```python
from build123d import *

# Parameters (mm, degrees)
BOSS_EXTRUDE1_DEPTH         = 50.8
FILLET1_R                   = 19.05
FILLET3_R                   = 3.81
F_1_4_20_TAPPED_HOLE1_D     = 5.1054
F_1_4_20_TAPPED_HOLE1_DEPTH = 19.05
F_1_4_20_TAPPED_HOLE1_TIP   = 1.533816902
M3_CLEARANCE_HOLE2_D        = 3.4


with BuildPart() as part:
    # Sketch1 → Boss-Extrude1 (new body)
    with BuildSketch(Plane.XY):
        Polygon((-20.6375, 0), (20.6375, 0), (20.6375, 6.35), (20.6375, 31.75), (12.7, 31.75), (12.7, 6.35), (-12.7, 6.35), (-12.7, 31.75), (-20.6375, 31.75), (-20.6375, 6.35), align=None)
    extrude(amount=BOSS_EXTRUDE1_DEPTH)

    # Fillet1
    fillet1_edges = [part.edges().sort_by_distance(p)[0] for p in [
        (-16.66875, 31.75, 0),
        (16.66875, 31.75, 50.8),
        (16.66875, 31.75, 0),
        (-16.66875, 31.75, 50.8),
    ]]
    fillet(fillet1_edges, radius=FILLET1_R)

    # Fillet3
    fillet3_edges = [part.edges().sort_by_distance(p)[0] for p in [
        (-12.7, 6.35, 25.4),
        (12.7, 6.35, 25.4),
    ]]
    fillet(fillet3_edges, radius=FILLET3_R)

    # 1/4-20 Tapped Hole1
    with Locations(Plane(origin=(0, 0, 0), x_dir=(-1, 0, 0), z_dir=(0, -1, 0))):
        with Locations((-16.66875, -3.96875), (16.66875, -3.96875), (16.66875, -46.83125), (-16.66875, -46.83125)):
            Hole(F_1_4_20_TAPPED_HOLE1_D / 2, depth=F_1_4_20_TAPPED_HOLE1_DEPTH)
            with Locations((0, 0, -(F_1_4_20_TAPPED_HOLE1_DEPTH + F_1_4_20_TAPPED_HOLE1_TIP / 2))):  # 118° drill point
                Cone(0, F_1_4_20_TAPPED_HOLE1_D / 2, F_1_4_20_TAPPED_HOLE1_TIP, mode=Mode.SUBTRACT)

    # M3 Clearance Hole2 (through all)
    with Locations(Plane(origin=(20.6375, 0, 0), x_dir=(0, 0, -1), z_dir=(1, 0, 0))):
        with Locations((-23.391086867, 19.05)):
            Hole(M3_CLEARANCE_HOLE2_D / 2)


solid = part.part
```
Input: part model. Units: mm. Frame: model coordinates. A direction names the side the tool comes from. Coordinates: 2 decimals unless noted, no trailing zeros. Loops run counter-clockwise (first coordinate to the right, second up) from the corner with the lowest first, then second, coordinate; pieces in that order, holes last. Notation, with made-up numbers: M 7.5,-40 L 37.5,-40 A19 ccw 37.5,-15 Z; hole C 89,18 d8. An arc over 180 degrees is marked long. One line per item, written item: value.
(1) Section B-B (y = 7). Output: boundary loops of the cut face in (x, z), and give its area (3 significant figures).
Filled in:
outline: M -20.64,0 L -11.02,0 L -11.02,50.8 L -20.64,50.8 Z; M 11.02,0 L 20.64,0 L 20.64,50.8 L 11.02,50.8 Z; hole C -16.67,3.97 d5.11; hole C -16.67,46.83 d5.11; hole C 16.67,3.97 d5.11; hole C 16.67,46.83 d5.11
area: 895 mm^2
(2) Section A-A (y = 11.5). Output: boundary loops of the cut face in (x, z).
Filled in:
outline: M -20.64,0 L -12.7,0 L -12.7,50.8 L -20.64,50.8 Z; M 12.7,0 L 20.64,0 L 20.64,50.8 L 12.7,50.8 Z; hole C -16.67,3.97 d5.11; hole C -16.67,46.83 d5.11; hole C 16.67,3.97 d5.11; hole C 16.67,46.83 d5.11
(3) Pin query (flat end, axial travel): pin 1 (4.5 mm diameter, centred on x = -16.67, z = 46.83, fed in from -Y); pin 2 (5 mm diameter, centred on x = -7.5, z = 37, fed in from +Y); pin 3 (8 mm diameter, centred on x = 16.67, z = 3.97, fed in from +Y); pin 4 (3 mm diameter, centred on y = 19.05, z = 23.39, fed in from -X). Return the tip coordinate at first contact, or that it passes through.
Filled in:
pin 1: y = 19.23
pin 2: y = 6.52
pin 3: y = 28.2
pin 4: through
(4) Line query: line 1 along X through (y, z) = (16, 16); line 2 along Z through (x, y) = (-17.5, 2.5); line 3 along Z through (x, y) = (-15, 19). Output: solid intervals per line, ascending. Write a range as from..to.
Filled in:
line 1: -20.64..-12.7, 12.7..20.64
line 2: 0..1.56, 6.38..44.42, 49.24..50.8
line 3: 1.07..2.04, 5.9..21.69, 25.09..44.9, 48.76..49.73
(5) Section C-C (z = 22.5). Output: boundary loops of the cut face in (x, y), and give its area (3 significant figures).
Filled in:
outline: M -20.64,0 L 20.64,0 L 20.64,17.6 L 12.7,17.6 L 12.7,10.16 A3.81 cw 8.89,6.35 L -8.89,6.35 A3.81 cw -12.7,10.16 L -12.7,17.6 L -20.64,17.6 Z; M -20.64,20.5 L -12.7,20.5 L -12.7,31.75 L -20.64,31.75 Z; M 12.7,20.5 L 20.64,20.5 L 20.64,31.75 L 12.7,31.75 Z
area: 626 mm^2
(6) Section D-D (x = 0). Output: boundary loops of the cut face in (y, z), and give its area (3 significant figures).
Filled in:
outline: M 0,0 L 6.35,0 L 6.35,50.8 L 0,50.8 Z
area: 323 mm^2
(7) Reachability of faces 4 (the flat face through (-20.638, 16, 25)), 5 (the flat face through (0, 6.35, 25)), 6 (the cylindrical face through (-18.55, 9.658, 2.244)) from +Z, -Z, +X, -X, +Y, -Y: full face, straight path, thin tool, end or side. Return the list, or none.
Filled in:
face 4: +Z, -Z, -X, +Y, -Y
face 5: +Z, -Z, +Y
face 6: -Y
(8) Pull-direction query (Z, two-part tool) for faces 1 (the cylindrical face through (-18.55, 9.658, 45.106)), 2 (the flat face through (0, 5, 50.8)), 3 (the flat face through (0, 5, 0)); classes: +Z half, -Z half, draft (parallel to the pull), parting line (faces both ways), or undercut.
Filled in:
face 1: undercut
face 2: +Z half
face 3: -Z half
